Autodesk Inventor part; units mm, degrees
ref_plane "YZ Plane" through (0, 0, 0) normal (1, 0, 0) x (0, 1, 0)
ref_plane "XZ Plane" through (0, 0, 0) normal (0, 1, 0) x (-1, 0, 0)
ref_plane "XY Plane" through (0, 0, 0) normal (0, 0, 1) x (1, 0, 0)
sketch "Sketch1" plane through (0, 0, 0) normal (0, 0, 1) x (1, 0, 0)
  circle A0 centre (0, 5) radius 7.5
  line L0 (42.7333, 18.5) -> (-42.7333, 18.5)
  line L1 (-42.7333, -29) -> (42.7333, -29)
  circle A1 centre (18.5, 5) radius 2.25
  circle A2 centre (-18.5, 5) radius 2.25
  circle A3 centre (30.8333, 5) radius 3.9
  circle A4 centre (-30.8333, 5) radius 3.9
  line L2 (42.7333, 18.5) -> (42.7333, -29)
  line L3 (-42.7333, -29) -> (-42.7333, 18.5)
  circle A5 centre (0, 5) radius 13.5 construction
  line L4 (0, 41.7106) -> (0, -39.2634) construction
  dimension "d2" = 4.5
  dimension "d3" = 4.5
  dimension "d4" = 7.8
  dimension "d5" = 7.8
  dimension "d48" = 47.5
  dimension "d58" = 15
  dimension "d63" = 27
  dimension "d75" = 34
  dimension "d76" = 30.8333
  dimension "d77" = 85.4667
  dimension "d93" = 47.5
extrude "Extrusion1" add sketch "Sketch1" against normal blind 3 contours A0 | L2 L1 L3 L0 | A1 | A2
sketch "Sketch4" plane through (0, 0, 0) normal (0, 0, 1) x (1, 0, 0)
  line L0 (42.7333, 18.5) -> (39.7333, 18.5)
  line L1 (-42.7333, 18.5) -> (-39.7333, 18.5)
  line L2 (42.7333, -29) -> (21.3667, -29)
  line L3 (21.3667, -26) -> (39.7333, -26)
  line L4 (-42.7333, -29) -> (-21.3667, -29)
  line L5 (-21.3667, -29) -> (-21.3667, -26)
  line L6 (-21.3667, -26) -> (-39.7333, -26)
  line L7 (-42.7333, -23) -> (-42.7333, -29)
  line L8 (42.7333, 18.5) -> (39.7333, 18.5)
  line L9 (39.7333, 18.5) -> (39.7333, 2.6667)
  line L10 (39.7333, 2.6667) -> (42.7333, 2.6667)
  line L11 (42.7333, 2.6667) -> (42.7333, 18.5)
  line L12 (39.7333, -26) -> (39.7333, -13.1667)
  line L13 (39.7333, -13.1667) -> (42.7333, -13.1667)
  line L14 (-42.7333, 2.6667) -> (-39.7333, 2.6667)
  line L15 (-39.7333, 2.6667) -> (-39.7333, 18.5)
  line L16 (-39.7333, 18.5) -> (-42.7333, 18.5)
  line L17 (-42.7333, 18.5) -> (-42.7333, 2.6667)
  line L18 (-42.7333, -29) -> (-39.7333, -29)
  line L19 (-39.7333, -26) -> (-39.7333, -13.1667)
  line L20 (-39.7333, -13.1667) -> (-42.7333, -13.1667)
  line L21 (-42.7333, -13.1667) -> (-42.7333, -29)
  line L22 (21.3667, -29) -> (21.3667, -26)
  line L23 (-21.3667, -23) -> (-21.3667, -29)
  line L24 (-42.7333, 18.5) -> (-39.7333, 18.5)
  line L25 (-42.7333, -29) -> (42.7333, -29)
  line L26 (42.7333, 18.5) -> (-42.7333, 18.5)
  line L27 (50.1623, -5.25) -> (-50.4474, -5.25) construction
  line L28 (42.7333, -29) -> (42.7333, 18.5)
  line L29 (42.7333, -3.75) -> (34.7333, -3.75)
  line L30 (34.7333, -3.75) -> (34.7333, -6.75)
  line L31 (34.7333, -6.75) -> (42.7333, -6.75)
  line L32 (42.7333, -6.75) -> (42.7333, -3.75)
  circle A0 centre (0, 5) radius 13.5 construction
  circle A1 centre (0, 5) radius 7.5 construction
  line L33 (42.7333, -2.6) -> (39.7333, -2.6)
  line L34 (39.7333, -2.6) -> (39.7333, -7.9)
  line L35 (39.7333, -7.9) -> (42.7333, -7.9)
  line L36 (42.7333, -7.9) -> (42.7333, -2.6)
  line L37 (35.3333, -2.6) -> (37.7333, -2.6)
  line L38 (37.7333, -2.6) -> (37.7333, -7.9)
  line L39 (37.7333, -7.9) -> (35.3333, -7.9)
  line L40 (35.3333, -7.9) -> (35.3333, -2.6)
  line L41 (0, 33.7344) -> (0, -36.9537) construction
  line L42 (-42.7333, 18.5) -> (-42.7333, -29)
  line L43 (-42.7333, -3.75) -> (-34.7333, -3.75)
  line L44 (-34.7333, -3.75) -> (-34.7333, -6.75)
  line L45 (-34.7333, -6.75) -> (-42.7333, -6.75)
  line L46 (-42.7333, -6.75) -> (-42.7333, -3.75)
  line L47 (-42.7333, -2.6) -> (-39.7333, -2.6)
  line L48 (-39.7333, -2.6) -> (-39.7333, -7.9)
  line L49 (-39.7333, -7.9) -> (-42.7333, -7.9)
  line L50 (-42.7333, -7.9) -> (-42.7333, -2.6)
  line L51 (-35.3333, -2.6) -> (-37.7333, -2.6)
  line L52 (-37.7333, -2.6) -> (-37.7333, -7.9)
  line L53 (-37.7333, -7.9) -> (-35.3333, -7.9)
  line L54 (-35.3333, -7.9) -> (-35.3333, -2.6)
  line L55 (42.7333, -29) -> (-42.7333, -29)
  line L56 (-1.5, -29) -> (1.5, -29)
  line L57 (1.5, -29) -> (1.5, -21)
  line L58 (1.5, -21) -> (-1.5, -21)
  line L59 (-1.5, -21) -> (-1.5, -29)
  line L60 (-2.65, -29) -> (2.65, -29)
  line L61 (2.65, -29) -> (2.65, -26)
  line L62 (2.65, -26) -> (-2.65, -26)
  line L63 (-2.65, -26) -> (-2.65, -29)
  line L64 (-2.65, -21.6) -> (2.65, -21.6)
  line L65 (2.65, -21.6) -> (2.65, -24)
  line L66 (2.65, -24) -> (-2.65, -24)
  line L67 (-2.65, -24) -> (-2.65, -21.6)
  line L68 (31.3, 16) -> (24.0167, 16) construction
  line L69 (11.4333, 16) -> (11.4333, 13) construction
  line L70 (11.4333, 13) -> (18.7167, 13) construction
  line L71 (31.3, 13) -> (31.3, 16) construction
  circle A2 centre (30.8333, 5) radius 3.9
  line L72 (21.3667, 17.602) -> (21.3667, 7.8585) construction
  line L73 (18.7167, 16) -> (24.0167, 16) construction
  line L74 (24.0167, 16) -> (24.0167, 13) construction
  line L75 (24.0167, 13) -> (18.7167, 13) construction
  line L76 (18.7167, 13) -> (18.7167, 16) construction
  line L77 (18.7167, 16) -> (11.4333, 16) construction
  line L78 (24.0167, 13) -> (31.3, 13) construction
  circle A3 centre (21.3667, 14.5) radius 1.4
  line L79 (-31.3, 16) -> (-24.0167, 16) construction
  line L80 (-11.4333, 16) -> (-11.4333, 13) construction
  line L81 (-11.4333, 13) -> (-18.7167, 13) construction
  line L82 (-31.3, 13) -> (-31.3, 16) construction
  line L83 (-24.0167, 16) -> (-24.0167, 13) construction
  line L84 (-18.7167, 13) -> (-18.7167, 16) construction
  line L85 (-18.7167, 16) -> (-11.4333, 16) construction
  line L86 (-24.0167, 13) -> (-31.3, 13) construction
  circle A4 centre (-21.3667, 14.5) radius 1.4
  line L87 (42.7333, 18.5) -> (42.7333, -29)
  line L88 (42.7333, -13.1667) -> (42.7333, -29)
  line L89 (18.7077, 16) -> (18.7077, 13)
  line L90 (19.8577, 13) -> (18.7077, 13)
  line L91 (19.8577, 16) -> (19.8577, 13)
  line L92 (18.7077, 16) -> (19.8577, 16)
  line L93 (11.4247, 16) -> (18.7077, 16)
  line L94 (11.4247, 13) -> (11.4247, 16)
  line L95 (11.4247, 13) -> (-11.4243, 13)
  line L96 (-11.4243, 16) -> (-11.4243, 13)
  line L97 (-18.7073, 16) -> (-11.4243, 16)
  line L98 (-18.7073, 13) -> (-18.7073, 16)
  line L99 (-18.7073, 13) -> (-19.8573, 13)
  line L100 (-19.8573, 13) -> (-19.8573, 16)
  line L101 (-19.8573, 16) -> (-18.7073, 16)
  line L102 (18.7077, 13) -> (11.4247, 13)
  line L103 (-11.4243, 16) -> (11.4247, 16)
  line L104 (-11.4243, 13) -> (-18.7073, 13)
  line L105 (24.0077, 13) -> (24.0077, 16)
  line L106 (22.8577, 16) -> (24.0077, 16)
  line L107 (22.8577, 13) -> (22.8577, 16)
  line L108 (24.0077, 13) -> (22.8577, 13)
  line L109 (31.2907, 13) -> (24.0077, 13)
  line L110 (31.2907, 16) -> (31.2907, 13)
  line L111 (31.2907, 16) -> (42.7337, 16)
  line L112 (42.7337, 16) -> (42.7337, 13)
  line L113 (42.7337, 13) -> (31.2907, 13)
  line L114 (24.0077, 16) -> (31.2907, 16)
  line L115 (-42.7333, 13) -> (-42.7333, 16)
  line L116 (-42.7333, 16) -> (-31.2903, 16)
  line L117 (-31.2903, 13) -> (-31.2903, 16)
  line L118 (-24.0073, 13) -> (-31.2903, 13)
  line L119 (-24.0073, 16) -> (-24.0073, 13)
  line L120 (-24.0073, 16) -> (-22.8573, 16)
  line L121 (-22.8573, 16) -> (-22.8573, 13)
  line L122 (-22.8573, 13) -> (-24.0073, 13)
  line L123 (-31.2903, 13) -> (-42.7333, 13)
  line L124 (-31.2903, 16) -> (-24.0073, 16)
  dimension "d25" = 3
  dimension "d26" = 3
  dimension "d33" = 15.8333
  dimension "d59" = 8
  dimension "d60" = 3
  dimension "d61" = 47.5
  dimension "d62" = 27
  dimension "d65" = 5.3
  dimension "d66" = 2.4
  dimension "d68" = 5
  dimension "d69" = 3
  dimension "d70" = 8
  dimension "d71" = 5.3
  dimension "d74" = 5
  dimension "d78" = 3
  dimension "d81" = 3
  dimension "d82" = 11
  dimension "d83" = 19.8667
  dimension "d85" = 79.4667
  dimension "d86" = 85.4667
  dimension "d87" = 3
  dimension "d88" = 5.3
  dimension "d89" = 2.8
  dimension "d91" = 15.8333
  dimension "d92" = 21.3667
  dimension "d94" = 2.4
  dimension "d95" = 2.4
extrude "Extrusion2" cut sketch "Sketch4" against normal through all contours L11 L111 L9 L0 | L11 L113 L9 L111 | L15 L116 L17 L1 | L11 L10 L9 L113 | L110 L109 L105 L114 | L15 L123 L17 L116 | L15 L14 L17 L123 | L124 L119 L118 L117 | L28 L29 L34 L33 | L28 L31 L34 L29 | L28 L35 L34 L31 | L34 L31 L38 L29 | L47 L48 L43 L42 | L38 L31 L40 L29 | L29 L40 L37 L38 | L43 L48 L45 L42 | L28 L2 L22 L3 L12 L13 | L38 L39 L40 L31 | L40 L31 L30 L29 | L45 L48 L49 L42 | L43 L52 L45 L48 | L52 L51 L54 L43 | L43 L54 L45 L52 | L20 L19 L6 L5 L4 L7 L21 | L45 L54 L53 L52 | L43 L44 L45 L54 | L25 L57 L62 L61 | L25 L59 L62 L57 | L25 L63 L62 L59 | L62 L59 L66 L57 | L66 L59 L64 L57 | L57 L64 L65 L66 | L66 L67 L64 L59 | L64 L59 L58 L57 | A3 | A4 | L89 L102 L94 L93 | L96 L104 L98 L97
equation "\"d48\" = d75 + 0.5 * d63"
equation "\"d33\" = 0.333333 * d61"
properties part number "X-Anchor_Back"
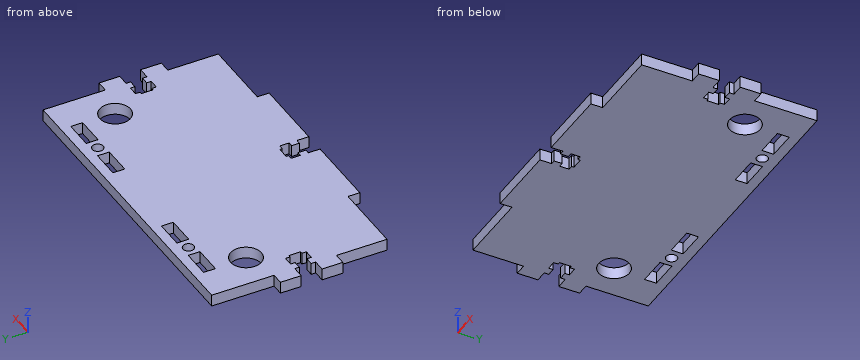
Geometry check sheet. Reference: the model listing, model coordinates, mm. Round coordinates to 2 decimals unless told otherwise and drop trailing zeros. Write each loop counter-clockwise with the first axis right and the second up, starting at its lowest first coordinate (ties: lowest second). Pieces come first, ordered by that corner, then holes.
Item 1: Section check A-A (x = -28). Record the boundary of the cut face in (y, z).
Determined:
outline: (-26, -3) - (2.32, -3) - (2.32, 0) - (-26, 0) - close; (7.68, -3) - (13, -3) - (13, 0) - (7.68, 0) - close; (16, -3) - (18.5, -3) - (18.5, 0) - (16, 0) - close
Item 2: Section check D-D (z = -1.45). Give the number of separate pieces and of enclosed holes in the cut face, plus the area to 3 significant figures.
Determined:
separate pieces: 1
enclosed holes: 8
area: 3,450 mm2
Item 3: Section check C-C (y = 5). Record the boundary of the cut face in (x, z).
Determined:
outline: (-39.73, -3) - (-34.73, -3) - (-34.73, 0) - (-39.73, 0) - close; (-26.93, -3) - (26.93, -3) - (26.93, 0) - (-26.93, 0) - close; (34.73, -3) - (39.73, -3) - (39.73, 0) - (34.73, 0) - close
Item 4: Section check B-B (y = 14.5). Record the boundary of the cut face in (x, z).
Determined:
outline: (-39.73, -3) - (-31.29, -3) - (-31.29, 0) - (-39.73, 0) - close; (-24.01, -3) - (-22.77, -3) - (-22.77, 0) - (-24.01, 0) - close; (-19.97, -3) - (-18.71, -3) - (-18.71, 0) - (-19.97, 0) - close; (-11.42, -3) - (11.42, -3) - (11.42, 0) - (-11.42, 0) - close; (18.71, -3) - (19.97, -3) - (19.97, 0) - (18.71, 0) - close; (22.77, -3) - (24.01, -3) - (24.01, 0) - (22.77, 0) - close; (31.29, -3) - (39.73, -3) - (39.73, 0) - (31.29, 0) - close
Item 5: Material ranges on line 1 along X through (y, z) = (-7, -1.95); line 2 along Y through (x, z) = (36, -1.95); line 3 along Y through (x, z) = (-18, -1.2), recorded low to high.
Determined:
line 1: x = -39.73 to -37.73, -35.33 to 35.33, 37.73 to 39.73
line 2: y = -26 to -7.9, -2.6 to 18.5
line 3: y = -29 to 13, 16 to 18.5
Item 6: Go/stop test with flat-tipped pins: pin 1 Ø0.6 at (x, z) = (2, -2) entering from -Y; pin 2 Ø0.9 at (y, z) = (14.5, -2) entering from +X; pin 3 Ø0.9 at (y, z) = (-28, -2) entering from +X. Record where each tip stops, or that it passes through.
Determined:
pin 1: stops at y = -26
pin 2: stops at x = 39.73
pin 3: stops at x = 21.37
